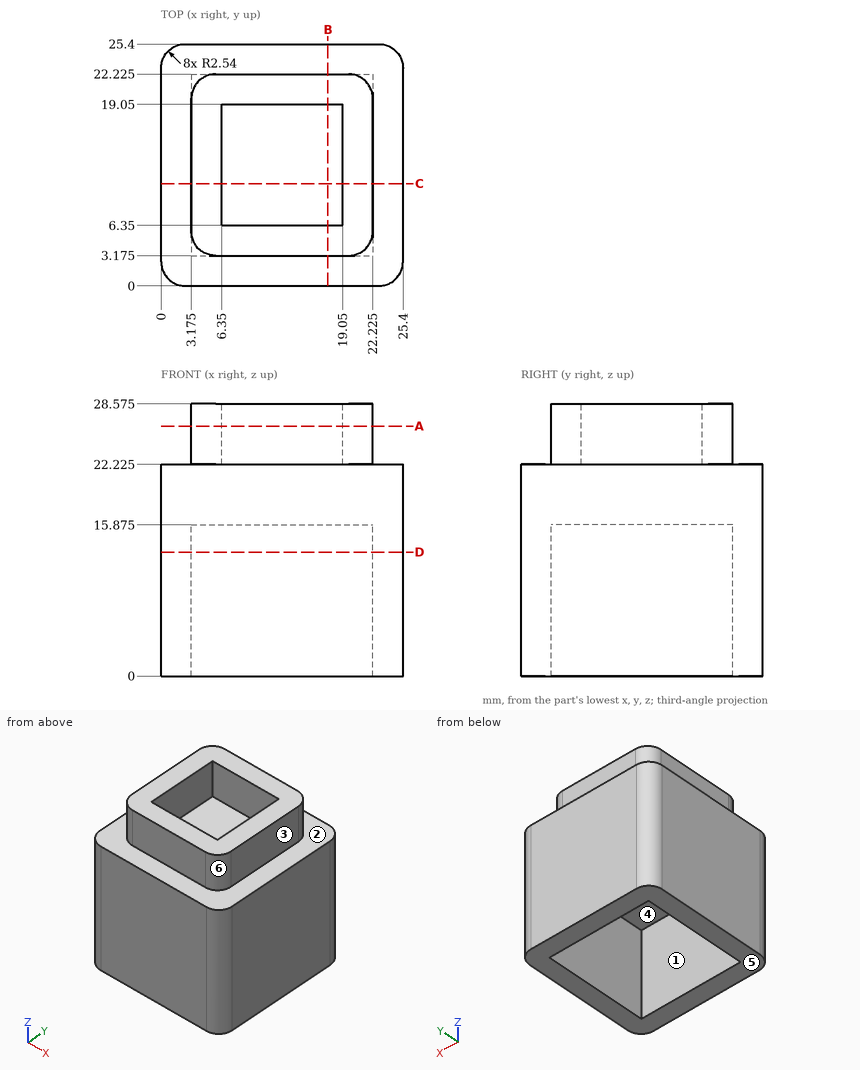
Print and shaded views of the part. All mm, measured from the part's lowest x, y and z. A direction names the side the tool comes from. Give positions to 0.01 mm unless a question says otherwise; leave off trailing zeros. Write each loop counter-clockwise with the first axis right and the second up, starting at its lowest first coordinate (ties: lowest second). Pieces come first, ordered by that corner, then holes. Notation, with made-up numbers: (1, 41.5) - (33, 41.5) arc R16 cw to (33, 64.5) - close; hole circle Ø4 at (26, -39). An arc over 180 degrees is marked (long way). One line per question, with ' | ' between items. Start each with the question number.
(1) Wall check: line 1 along X through (y, z) = (20.5, 2) (3 decimals); line 2 along X through (y, z) = (9, 23.25) (3 decimals). Give the ranges that are in metal, low to high. Write a range as from..to.
(2) Slice it at B-B on x = 17.5. Write the cut outline in (y, z) (3 decimals), plus the area to 3 significant figures.
(3) Slice it at A-A on z = 26.25. Write the cut outline in (x, y) (3 decimals).
(4) Pin check, flat tips, straight feed: P1, Ø3, axis at x = 15, z = 25, coming from the -Y side (3 decimals); P2, Ø5.5, axis at x = 9, y = 13, coming from the -Z side (3 decimals); P3, Ø1.9, axis at x = 11, z = 25.5, coming from the +Y side (3 decimals). Stop position of each tip, or through.
(5) 3-axis set-ups, long thin cutter, end or side, ignore diameter. For the marked faces 1, 2 and 3: which of +Z, -Z, +X, -X, +Y, -Y reach the whole face in a straight line?
(6) Slice it at D-D on z = 13. Write the cut outline in (x, y) (3 decimals), plus the area to 3 significant figures.
(7) Two-plate mould, pull along Y, no slides. Class the marked faces 4, 5 and 6: +Y half, -Y half, draft (parallel to the pull), parting line (faces both ways), or undercut.
Results below:
1) line 1: 0..3.175, 22.225..25.4 | line 2: 3.175..6.35, 19.05..22.225
2) outline: (0, 0) - (3.175, 0) - (3.175, 15.875) - (22.225, 15.875) - (22.225, 0) - (25.4, 0) - (25.4, 22.225) - (22.225, 22.225) - (22.225, 28.575) - (19.05, 28.575) - (19.05, 22.225) - (6.35, 22.225) - (6.35, 28.575) - (3.175, 28.575) - (3.175, 22.225) - (0, 22.225) - close | area: 302 mm^2
3) outline: (3.175, 5.715) arc R2.54 ccw to (5.715, 3.175) - (19.685, 3.175) arc R2.54 ccw to (22.225, 5.715) - (22.225, 19.685) arc R2.54 ccw to (19.685, 22.225) - (5.715, 22.225) arc R2.54 ccw to (3.175, 19.685) - close; hole (6.35, 6.35) - (19.05, 6.35) - (19.05, 19.05) - (6.35, 19.05) - close
4) P1: y = 3.175 | P2: z = 15.875 | P3: y = 22.225
5) face 1: -Z | face 2: +Z | face 3: +Z, +X, +Y, -Y
6) outline: (0, 2.54) arc R2.54 ccw to (2.54, 0) - (22.86, 0) arc R2.54 ccw to (25.4, 2.54) - (25.4, 22.86) arc R2.54 ccw to (22.86, 25.4) - (2.54, 25.4) arc R2.54 ccw to (0, 22.86) - close; hole (3.175, 3.175) - (22.225, 3.175) - (22.225, 22.225) - (3.175, 22.225) - close | area: 277 mm^2
7) face 4: undercut | face 5: draft | face 6: -Y half
